The model under review builds one solid part; all positions refer to its coordinate system, in mm. Face numbers are marked on the shaded views. A direction names the side the tool comes from. Round coordinates to 2 decimals unless told otherwise and drop trailing zeros. Order: outer loops, then holes, each group sorted by start corner. A loop starts at its lowest first (then second) coordinate and runs counter-clockwise, first axis right, second up.
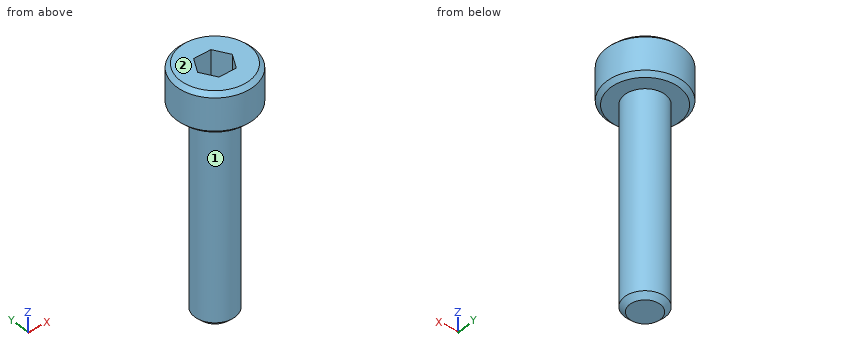
from build123d import *

# Parameters (mm, degrees)
CUT_EXTRUDE_1_DEPTH = 1.8


with BuildPart() as part:
    # Эскиз1 → Повернуть1 (revolve)
    with BuildSketch(Plane(origin=(0, 0, 0), x_dir=(1, 0, 0), z_dir=(0, 1, 0))):
        Polygon((0, 0), (1.7, 0), (1.9, 0.2), (1.9, 1.8), (1.7, 2), (1, 2), (1, 11.75), (0.75, 12), (0, 12), align=None)
    revolve(axis=Axis((0, 0, 0), (0, 0, -1)))

    # Эскиз2 → Вырез-Вытянуть1 (cut)
    with BuildSketch(Plane.XY):
        Polygon((0.866025404, 0), (0.433012702, 0.75), (-0.433012702, 0.75), (-0.866025404, 0), (-0.433012702, -0.75), (0.433012702, -0.75), align=None)
    extrude(amount=-CUT_EXTRUDE_1_DEPTH, mode=Mode.SUBTRACT)


solid = part.part
(1) Tool access review of the marked faces 1 and 2: name each direction out of +Z, -Z, +X, -X, +Y, -Y from which nothing blocks a thin tool from reaching the whole face with its end or side.
(2) To check wall thickness, follow L1, parallel to Z at x = -0.2, y = -0.5; L2, parallel to X at y = -0.9, z = -7; L3, parallel to Z at x = 0.55, y = -1.5. State the ranges of each line that lie inside material, in increasing order.
(3) We need section A-A (z = -1.5). Give the boundary of the cut face in (x, y), and give its area (3 significant figures).
(4) We need section B-B (x = 0). Give the boundary of the cut face in (y, z).
(5) Clearance check with flat-ended pins moving along their axes: P1, Ø2, axis at x = -0.5, z = -10.5, coming from the -Y side; P2, Ø2, axis at x = 0, z = -4.5, coming from the +Y side; P3, Ø1.5, axis at x = 1.5, y = 1.5, coming from the -Z side. State where each tip first meets the part, or that it passes through.
(6) We need section C-C (z = -2.75). Give the boundary of the cut face in (x, y), and give its area (3 significant figures).
Verdict:
1. face 1: -Z
1. face 2: +Z, +X, -X, +Y, -Y
2. L1: z = -12 to -1.8
2. L2: x = -0.44 to 0.44
2. L3: z = -2 to 0
3. outline: circle Ø3.8 at (0, 0); hole (-0.87, 0) - (-0.43, -0.75) - (0.43, -0.75) - (0.87, 0) - (0.43, 0.75) - (-0.43, 0.75) - close
3. area: 9.39 mm2
4. outline: (-1.9, -1.8) - (-1.7, -2) - (-1, -2) - (-1, -11.75) - (-0.75, -12) - (0.75, -12) - (1, -11.75) - (1, -2) - (1.7, -2) - (1.9, -1.8) - (1.9, -0.2) - (1.7, 0) - (0.75, 0) - (0.75, -1.8) - (-0.75, -1.8) - (-0.75, 0) - (-1.7, 0) - (-1.9, -0.2) - close
5. P1: stops at y = -1
5. P2: stops at y = 1
5. P3: stops at z = -2
6. outline: circle Ø2 at (0, 0)
6. area: 3.14 mm2
